Work out the finished part from the listing and answer in its coordinate system (mm). Face numbers are marked on the shaded views. Coordinates: 2 decimals unless noted, no trailing zeros. Loops run counter-clockwise (first coordinate to the right, second up) from the corner with the lowest first, then second, coordinate; pieces in that order, holes last. Notation, with made-up numbers: (-11, -40) -> (16, -40) arc R23 cw to (16, -19) -> close; hole circle Ø4 at (43.5, 83.25). An arc over 180 degrees is marked (long way). One line per question, with ' | ' between items.
```python
from build123d import *

# Parameters (mm, degrees)
ESQUISSE1_W                = 160
ESQUISSE1_H                = 100
ESQUISSE1_W_2              = 144
ESQUISSE1_H_2              = 90
PROFONDEUR_COUVERCLE_DEPTH = 15
ESQUISSE2_W                = 144
ESQUISSE2_H                = 90
PROFONDEUR_FOND_DEPTH      = 5
ESQUISSE3_W                = 24
ESQUISSE3_H                = 14
ECRAN_HELTEC_DEPTH         = 21


with BuildPart() as part:
    # Esquisse1 → profondeur couvercle (new body)
    with BuildSketch(Plane.XY):
        Rectangle(ESQUISSE1_W, ESQUISSE1_H)
        Rectangle(ESQUISSE1_W_2, ESQUISSE1_H_2, mode=Mode.SUBTRACT)
    extrude(amount=PROFONDEUR_COUVERCLE_DEPTH)

    # Esquisse2 → profondeur fond (add)
    with BuildSketch(Plane.XY):
        Rectangle(ESQUISSE2_W, ESQUISSE2_H)
    extrude(amount=PROFONDEUR_FOND_DEPTH)

    # Esquisse3 → ecran heltec (cut)
    with BuildSketch(Plane.XY):
        with Locations((48, -3)):
            Rectangle(ESQUISSE3_W, ESQUISSE3_H)
    extrude(amount=ECRAN_HELTEC_DEPTH, mode=Mode.SUBTRACT)


solid = part.part
```
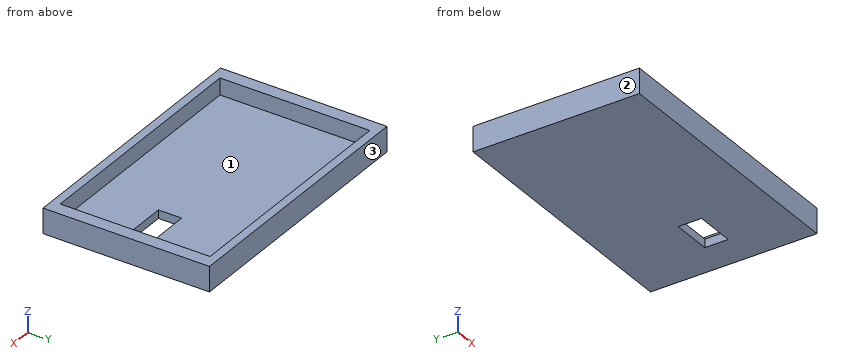
1) The mould has two halves that part along Y. Classify the marked faces 1, 2 and 3: released by +Y, released by -Y, zero draft, split by the parting line, or undercut.
Check values:
face 1: undercut | face 2: zero draft | face 3: released by +Y
2) Find section C-C (x = -26.5). Write down the section's boundary in (y, z).
Check values:
outline: (-50, 0) -> (50, 0) -> (50, 15) -> (45, 15) -> (45, 5) -> (-45, 5) -> (-45, 15) -> (-50, 15) -> close
3) Find the intervals of material crossed by line 1 along X through (y, z) = (-19.5, 13.5); line 2 along Y through (x, z) = (47, 12); line 3 along X through (y, z) = (3, 3.25), in increasing order.
Check values:
line 1: x = -80 to -72, 72 to 80 | line 2: y = -50 to -45, 45 to 50 | line 3: x = -80 to 36, 60 to 80
4) Find section A-A (x = 55). Write down the section's boundary in (y, z), plus the area to 3 significant figures.
Check values:
outline: (-50, 0) -> (-10, 0) -> (-10, 5) -> (-45, 5) -> (-45, 15) -> (-50, 15) -> close; (4, 0) -> (50, 0) -> (50, 15) -> (45, 15) -> (45, 5) -> (4, 5) -> close | area: 530 mm^2
5) A flat-ended cylindrical pin translates along its axis: pin 1 (1.5 mm diameter, centred on x = 20.5, y = -38.5, fed in from +Z). Find the tip coordinate at first contact, or state that the pin passes through.
Check values:
pin 1: stops at z = 5
6) Find section B-B (z = 8.5). Write down the section's boundary in (x, y).
Check values:
outline: (-80, -50) -> (80, -50) -> (80, 50) -> (-80, 50) -> close; hole (-72, -45) -> (72, -45) -> (72, 45) -> (-72, 45) -> close
7) Find section D-D (y = 30). Write down the section's boundary in (x, z).
Check values:
outline: (-80, 0) -> (80, 0) -> (80, 15) -> (72, 15) -> (72, 5) -> (-72, 5) -> (-72, 15) -> (-80, 15) -> close
